from build123d import *

# Parameters (mm, degrees)
F1_DEPTH = 50.8
F2_R     = 1.905
F3_DEPTH = 17.78
F6_DEPTH = 25.4
F8_DEPTH = 25.4
F4_R     = 1.905
F9_DEPTH = 17.78


with BuildPart() as f1:
    # F0 (on Front) → F1 (new body)
    with BuildSketch(Plane.XZ):
        Polygon((-9.1096315365, 61.225563957), (-19.2696315365, 61.225563957), (-19.2696315365, 48.525563957), (-16.9836315365, 48.525563957), (-16.9836315365, 32.015563957), (-14.1896315365, 32.015563957), (-11.3956315365, 32.015563957), (-11.3956315365, 48.525563957), (-9.1096315365, 48.525563957), align=None)
        Polygon((-14.1896315365, 32.015563957), (-16.9836315365, 32.015563957), (-49.3125535723, -0.3133580789), (-47.0674895421, -2.5584221091), (-14.1896315365, 30.3194358965), align=None)
        Polygon((-11.3956315365, 32.015563957), (-14.1896315365, 32.015563957), (-14.1896315365, 30.3194358965), (18.6882264691, -2.5584221091), (20.9332904994, -0.3133580789), align=None)
    extrude(amount=F1_DEPTH)

    # F2 (on face) → F3 (cut)
    with BuildSketch(Plane(origin=(0, 0, 0), x_dir=(-1, 0, 0), z_dir=(0, 1, 0))):
        with Locations((14.1358394176, 55.2771948278)):
            Circle(F2_R)
    extrude(amount=-F3_DEPTH, mode=Mode.SUBTRACT)

    # F5 (on face) → F6 (join)
    with BuildSketch(Plane(origin=(10.3099662102, 0, 10.3099662102), x_dir=(0.7071067812, 0, -0.7071067812), z_dir=(0.7071067812, 0, 0.7071067812))):
        with BuildLine():
            Line((-7.8363507129, -25.4), (-7.8363507129, -23.8125))
            ThreePointArc((-7.8363507129, -23.8125), (-8.958882728, -24.2774679849), (-9.4238507129, -25.4))
            Line((-9.4238507129, -25.4), (-7.8363507129, -25.4))
        make_face()
        with BuildLine():
            Line((-7.8363507129, -25.4), (-6.2488507129, -25.4))
            ThreePointArc((-6.2488507129, -25.4), (-6.7138186977, -24.2774679849), (-7.8363507129, -23.8125))
            Line((-7.8363507129, -23.8125), (-7.8363507129, -25.4))
        make_face()
        with BuildLine():
            ThreePointArc((-9.4238507129, -25.4), (-8.958882728, -26.5225320151), (-7.8363507129, -26.9875))
            Line((-7.8363507129, -26.9875), (-7.8363507129, -25.4))
            Line((-7.8363507129, -25.4), (-9.4238507129, -25.4))
        make_face()
        with BuildLine():
            ThreePointArc((-7.8363507129, -26.9875), (-6.7138186977, -26.5225320151), (-6.2488507129, -25.4))
            Line((-6.2488507129, -25.4), (-7.8363507129, -25.4))
            Line((-7.8363507129, -25.4), (-7.8363507129, -26.9875))
        make_face()
    extrude(amount=F6_DEPTH)

    # F7 (on face) → F8 (join)
    with BuildSketch(Plane(origin=(-24.4995977467, 0, 24.4995977467), x_dir=(0, -1, 0), z_dir=(-0.7071067812, 0, 0.7071067812))):
        with BuildLine():
            ThreePointArc((26.9875, -12.2308186511), (26.5225320151, -11.108286636), (25.4, -10.6433186511))
            Line((25.4, -10.6433186511), (25.4, -12.2308186511))
            Line((25.4, -12.2308186511), (26.9875, -12.2308186511))
        make_face()
        with BuildLine():
            Line((26.9875, -12.2308186511), (25.4, -12.2308186511))
            Line((25.4, -12.2308186511), (25.4, -13.8183186511))
            ThreePointArc((25.4, -13.8183186511), (26.5225320151, -13.3533506663), (26.9875, -12.2308186511))
        make_face()
        with BuildLine():
            Line((25.4, -12.2308186511), (23.8125, -12.2308186511))
            ThreePointArc((23.8125, -12.2308186511), (24.2774679849, -13.3533506663), (25.4, -13.8183186511))
            Line((25.4, -13.8183186511), (25.4, -12.2308186511))
        make_face()
        with BuildLine():
            Line((25.4, -12.2308186511), (25.4, -10.6433186511))
            ThreePointArc((25.4, -10.6433186511), (24.2774679849, -11.108286636), (23.8125, -12.2308186511))
            Line((23.8125, -12.2308186511), (25.4, -12.2308186511))
        make_face()
    extrude(amount=F8_DEPTH)

    # F4 (on face) → F9 (cut)
    with BuildSketch(Plane.XZ.offset(50.8)):
        with Locations((-13.9896953478, 55.213548243)):
            Circle(F4_R)
    extrude(amount=-F9_DEPTH, mode=Mode.SUBTRACT)


solid = f1.part
The model under review builds one solid part; all positions refer to its coordinate system, in mm. A direction names the side the tool comes from. Round coordinates to 2 decimals unless told otherwise and drop trailing zeros. Loops run counter-clockwise (first coordinate to the right, second up) from the corner with the lowest first, then second, coordinate; pieces in that order, holes last. Notation, with made-up numbers: (87.5, 63.25) -> (143.5, 63.25) arc R33 cw to (143.5, 92.25) -> close; hole circle Ø1 at (86, 72.25). An arc over 180 degrees is marked (long way). One line per question, with ' | ' between items. Start each with the question number.
Item 1: Add section B-B, the plane y = -29.5. Write out the cut boundary in (x, z).
Item 2: Add section D-D, the plane x = -25. Write out the cut boundary in (y, z).
Item 3: Machinability: for faces 4 (the face through (-15.16, -8.766, 56.883)), 5 (the face through (-30.86, -25.04, 13.65)), 6 (the face through (-14, -33.02, 55)), 7 (the face through (-18, -25, 48.526)), which of the approach directions +Z, -Z, +X, -X, +Y, -Y give a long, thin tool a straight path to every point of the face, cutting with its end or side? Answer none if there is none.
Item 4: Draft analysis for pull direction X (two halves, no side actions). For faces 1 (the face through (22.71, -25.38, 33.83)), 2 (the face through (-14, -17.78, 55)), 3 (the face through (-12, 0, 29)), state which applies: +X half, -X half, draft (parallel to the pull), parting line (faces both ways), or undercut.
Item 5: Add section C-C, the plane y = -15. Write out the cut boundary in (x, z) (3 decimals), then the cut area to 3 significant figures.
Item 6: For pin 1 (12 mm diameter, centred on x = -6, y = -44, fed in from -Z); pin 2 (5 mm diameter, centred on x = -20.5, y = -14, fed in from +Z); pin 3 (2.5 mm diameter, centred on x = -14.14, z = 55.28, fed in from +Y); pin 4 (12 mm diameter, centred on y = -17, z = 33, fed in from +X), all flat-tipped, find the tip position at first contact; note any pin that passes through.
Item 7: Add section A-A, the plane z = 8. Write out the cut boundary in (x, y), then the cut area to 3 significant figures.
Item 8: Wall thickness on line 1 along X through (y, z) = (-26, 23.5); line 2 along X through (y, z) = (-25.5, 43); line 3 along X through (y, z) = (-43, 14.5): over which ranges is each line inside the solid? List them lowest first. Write a range as [from, to].
Return value:
1) outline: (-49.31, -0.31) -> (-47.07, -2.56) -> (-14.19, 30.32) -> (18.69, -2.56) -> (20.93, -0.31) -> (-11.4, 32.02) -> (-11.4, 48.53) -> (-9.11, 48.53) -> (-9.11, 61.23) -> (-19.27, 61.23) -> (-19.27, 48.53) -> (-16.98, 48.53) -> (-16.98, 32.02) -> close
2) outline: (-50.8, 19.51) -> (0, 19.51) -> (0, 24) -> (-50.8, 24) -> close
3) face 4: +Y | face 5: -Z, +Y, -Y | face 6: -Y | face 7: -X, +Y, -Y
4) face 1: +X half | face 2: undercut | face 3: draft
5) outline: (-49.313, -0.313) -> (-47.067, -2.558) -> (-14.19, 30.319) -> (18.688, -2.558) -> (20.933, -0.313) -> (-11.396, 32.016) -> (-11.396, 48.526) -> (-9.11, 48.526) -> (-9.11, 61.226) -> (-19.27, 61.226) -> (-19.27, 48.526) -> (-16.984, 48.526) -> (-16.984, 32.016) -> close; hole circle Ø3.81 at (-14.136, 55.277) | area: 507 mm2
6) pin 1: stops at z = 16.13 | pin 2: stops at z = 61.23 | pin 3: stops at y = -17.78 | pin 4: stops at x = -6.38
7) outline: (-41, -50.8) -> (-36.51, -50.8) -> (-36.51, 0) -> (-41, 0) -> close; (8.13, -50.8) -> (12.62, -50.8) -> (12.62, 0) -> (8.13, 0) -> close | area: 456 mm2
8) line 1: x = [-42.88, -38.72], [-25.5, -21.01], [-7.37, -2.88], [10.34, 14.5] | line 2: x = [-16.98, -11.4] | line 3: x = [-34.5, -30.01], [1.63, 6.12]
